Source: CAD feature listing. Evaluate the final solid. Frame: model axes, mm. A direction names the side the tool comes from. Round coordinates to 2 decimals unless told otherwise and drop trailing zeros. Write each loop counter-clockwise with the first axis right and the second up, starting at its lowest first coordinate (ties: lowest second). Pieces come first, ordered by that corner, then holes. Notation, with made-up numbers: M 51,66 L 71,66 A13 cw 71,80 Z; hole C 26,-33.75 d11. An arc over 180 degrees is marked long. Answer in a Markdown table with one row per item.
from build123d import *

# Parameters (mm, degrees)
F2_DEPTH = 20
F4_DEPTH = 220
F5_W     = 104
F5_H     = 90
F6_DEPTH = 40
F7_DEPTH = 25
F8_DEPTH = 20


with BuildPart() as f2:
    # F1 (on face) → F2 (new body)
    with BuildSketch(Plane.XY):
        Polygon((413, -75), (688, -75), (688, 440), (290, 440), (290, 406), (290, 141), (290, -75), align=None)
    extrude(amount=F2_DEPTH)

    # F3 (on face) → F4 (join)
    with BuildSketch(Plane.XY.offset(20)):
        Polygon((667, 406), (667, -54), (413, -54), (413, -75), (688, -75), (688, 406), (688, 440), (290, 440), (290, -75), (312, -75), (312, 43), (312, 124), (312, 406), align=None)
    extrude(amount=F4_DEPTH)

    # F5 (on face) → F6 (cut)
    with BuildSketch(Plane(origin=(0, 440, 0), x_dir=(-1, 0, 0), z_dir=(0, 1, 0))):
        with Locations((-443, 175)):
            Rectangle(F5_W, F5_H)
    extrude(amount=-F6_DEPTH, mode=Mode.SUBTRACT)

    # F7 (cut): a face of the model
    f7_faces = [f2.faces().sort_by_distance(p)[0] for p in [
        (487.8716275443, 172.9163497984, 20),
    ]]
    extrude(f7_faces, amount=-F7_DEPTH, mode=Mode.SUBTRACT)

    # F8 (add): a face of the model
    f8_faces = [f2.faces().sort_by_distance(p)[0] for p in [
        (550.5, -68.4913211786, 0),
    ]]
    extrude(f8_faces, amount=F8_DEPTH)


solid = f2.part
Q1. Section D-D (x = 484). Return loops of the section in (y, z).
Solutions:
| item | result |
|---|---|
| outline | M -75,-20 L -54,-20 L -54,240 L -75,240 Z; M 406,-20 L 440,-20 L 440,130 L 406,130 Z; M 406,220 L 440,220 L 440,240 L 406,240 Z |
Q2. Material intervals for probe 1 along Y at (x, z) = (434, 46); probe 2 along X at (y, z) = (80, 129); probe 3 along Y at (x, z) = (440, 146), sorted ascending.
Solutions:
| item | result |
|---|---|
| probe 1 | y = -75 to -54, 406 to 440 |
| probe 2 | x = 290 to 312, 667 to 688 |
| probe 3 | y = -75 to -54 |
Q3. Section A-A (y = 90.5). Return loops of the section in (x, z).
Solutions:
| item | result |
|---|---|
| outline | M 290,-20 L 312,-20 L 312,240 L 290,240 Z; M 667,-20 L 688,-20 L 688,240 L 667,240 Z |
Q4. Section C-C (z = 193). Return loops of the section in (x, y).
Solutions:
| item | result |
|---|---|
| outline | M 290,-75 L 312,-75 L 312,406 L 391,406 L 391,440 L 290,440 Z; M 413,-75 L 688,-75 L 688,440 L 495,440 L 495,406 L 667,406 L 667,-54 L 413,-54 Z |
Q5. Access query for faces 4 (the flat face through (391, 423, 174)), 5 (the flat face through (667, 179, 112)), 6 (the flat face through (495, 423, 174)). Directions: +Z, -Z, +X, -X, +Y, -Y. A direction counts if a zero-diameter tool reaches every point of the face in a straight line with its end or side. Return the directions, or none.
Solutions:
| item | result |
|---|---|
| face 4 | +Y, -Y |
| face 5 | +Z, -Z |
| face 6 | +Y |
Q6. Section B-B (x = 592). Return loops of the section in (y, z), and give its area (3 significant figures).
Solutions:
| item | result |
|---|---|
| outline | M -75,-20 L -54,-20 L -54,240 L -75,240 Z; M 406,-20 L 440,-20 L 440,240 L 406,240 Z |
| area | 14,300 mm2 |
Q7. Pull-direction query (Y, two-part tool) for faces 1 (the flat face through (549, -75, 112)), 2 (the flat face through (487, 406, 112)), 3 (the flat face through (444, 423, 130)); classes: pulls with the +Y half, pulls with the -Y half, needs draft (parallel to the pull), parting line crosses it, or undercut.
Solutions:
| item | result |
|---|---|
| face 1 | pulls with the -Y half |
| face 2 | undercut |
| face 3 | needs draft |
